The model under review builds one solid part; all positions refer to its coordinate system, in mm. A direction names the side the tool comes from. Coordinates: 2 decimals unless noted, no trailing zeros. Loops run counter-clockwise (first coordinate to the right, second up) from the corner with the lowest first, then second, coordinate; pieces in that order, holes last. Notation, with made-up numbers: M 52.25,28 L 86.25,28 A13 ccw 86.25,37 Z; hole C -7.75,57 d7. An arc over 180 degrees is marked long. Return JSON: item names as keys, results as strings.
```python
from build123d import *

# Parameters (mm, degrees)
SALIENTE_EXTRUIR1_DEPTH     = 46
CROQUIS3_W                  = 5
CROQUIS3_H                  = 17
CORTAR_EXTRUIR1_DEPTH       = 107
VACIADO1_T                  = -5
CORTAR_EXTRUIR3_DEPTH       = 5
CROQUIS7_W                  = 28.084979232
CROQUIS7_H                  = 13.64051807
CORTAR_EXTRUIR5_DEPTH       = 2
CROQUIS8_W                  = 84.286700134
CROQUIS8_H                  = 59.012293191
CORTAR_EXTRUIR6_DEPTH       = 50
CROQUIS9_W                  = 89.93795334
CROQUIS9_H                  = 8.49113686
CORTAR_EXTRUIR7_DEPTH       = 10
REDONDEO1_R                 = 2
REDONDEO2_R                 = 2
REDONDEO3_R                 = 2
CROQUIS10_W                 = 19.827227688
CROQUIS10_H                 = 42.140696998
CORTAR_EXTRUIR8_DEPTH       = 2
CROQUIS11_R                 = 2.017504942
CROQUIS11_R_2               = 1.891140859
CORTAR_EXTRUIR9_DEPTH       = 9
CROQUIS12_R                 = 2.25
CORTAR_EXTRUIR10_DEPTH      = 33
CORTAR_EXTRUIR11_START      = -3
CROQUIS13_R                 = 2.075
CORTAR_EXTRUIR11_DEPTH      = 7
CORTAR_EXTRUIR12_DEPTH      = 20
CORTAR_EXTRUIR12_DEPTH_BACK = 1
CORTAR_EXTRUIR12_START      = 10
CROQUIS14_R                 = 2.5
CROQUIS15_W                 = 7.96749323
CROQUIS15_H                 = 3.005999516
SALIENTE_EXTRUIR2_DEPTH     = 10
CROQUIS16_R                 = 1.5
CORTAR_EXTRUIR13_DEPTH      = 73
CROQUIS17_W                 = 124.159046256
CROQUIS17_H                 = 73.830112024
CORTAR_EXTRUIR14_DEPTH      = 2
CORTAR_EXTRUIR15_DEPTH      = 10
SALIENTE_EXTRUIR3_DEPTH     = 41
REDONDEO4_R                 = 10


with BuildPart() as part:
    # Croquis1 → Saliente-Extruir1 (new body)
    with BuildSketch(Plane.XY):
        Polygon((-50, -27.25), (-50, -29.825247619), (50, -29.825247619), (50, -27.25), (50, 27.25), (-50, 27.25), align=None)
    extrude(amount=SALIENTE_EXTRUIR1_DEPTH)

    # Croquis3 → Cortar-Extruir1 (cut)
    with BuildSketch(Plane.ZY.offset(50)):
        Polygon((46, 27.25), (5, 27.25), (11, 16.857695155), (46, 8.318575661), align=None)
        with Locations((2.5, 18.75)):
            Rectangle(CROQUIS3_W, CROQUIS3_H)
    extrude(amount=-CORTAR_EXTRUIR1_DEPTH, mode=Mode.SUBTRACT)

    # Vaciado1
    vaciado1_openings = [part.faces().sort_by_distance(p)[0] for p in [
        (0, -10.753335979, 46),
    ]]
    offset(amount=VACIADO1_T, openings=vaciado1_openings, kind=Kind.INTERSECTION)

    # Croquis5 → Cortar-Extruir3 (cut)
    with BuildSketch(Plane(origin=(0, 0, 0), x_dir=(-1, 0, 0), z_dir=(0, 0, -1))):
        Polygon((-44.96897667, -22.941518711), (-44.96897667, -34.965963837), (44.96897667, -34.965963837), (44.96897667, -22.941518711), (44.96897667, 22.941518711), (-44.96897667, 22.941518711), align=None)
    extrude(amount=-CORTAR_EXTRUIR3_DEPTH, mode=Mode.SUBTRACT)

    # Croquis7 → Cortar-Extruir5 (cut)
    with BuildSketch(Plane(origin=(0, 0, 0), x_dir=(-1, 0, 0), z_dir=(0, 0, -1))):
        Rectangle(CROQUIS7_W, CROQUIS7_H)
    extrude(amount=-CORTAR_EXTRUIR5_DEPTH, mode=Mode.SUBTRACT)

    # Croquis8 → Cortar-Extruir6 (cut)
    with BuildSketch(Plane(origin=(0, 0, 2), x_dir=(-1, 0, 0), z_dir=(0, 0, -1))):
        with Locations((0, -42.853406707)):
            Rectangle(CROQUIS8_W, CROQUIS8_H)
    extrude(amount=-CORTAR_EXTRUIR6_DEPTH, mode=Mode.SUBTRACT)

    # Croquis9 → Cortar-Extruir7 (cut)
    with BuildSketch(Plane(origin=(0, 0, 5), x_dir=(-1, 0, 0), z_dir=(0, 0, -1))):
        with Locations((0, 9.49556843)):
            Rectangle(CROQUIS9_W, CROQUIS9_H)
    extrude(amount=-CORTAR_EXTRUIR7_DEPTH, mode=Mode.SUBTRACT)

    # Redondeo1
    redondeo1_edges = [part.edges().sort_by_distance(p)[0] for p in [
        (-50, -29.825247619, 23),
        (42.143350067, -29.825247619, 25.5),
    ]]
    fillet(redondeo1_edges, radius=REDONDEO1_R)

    # Redondeo2
    redondeo2_edges = [part.edges().sort_by_distance(p)[0] for p in [
        (50, -29.825247619, 23),
    ]]
    fillet(redondeo2_edges, radius=REDONDEO2_R)

    # Redondeo3
    redondeo3_edges = [part.edges().sort_by_distance(p)[0] for p in [
        (-42.143350067, -29.825247619, 25.5),
    ]]
    fillet(redondeo3_edges, radius=REDONDEO3_R)

    # Croquis10 → Cortar-Extruir8 (cut)
    with BuildSketch(Plane(origin=(0, 13.586066701, 3.314658486), x_dir=(1, 0, 0), z_dir=(0, -0.9715041436001179, -0.237022570587279))):
        with Locations((13.913613844, 22.867026133)):
            Rectangle(CROQUIS10_W, CROQUIS10_H)
        with Locations((-13.913613844, 22.867026133)):
            Rectangle(CROQUIS10_W, CROQUIS10_H)
    extrude(amount=-CORTAR_EXTRUIR8_DEPTH, mode=Mode.SUBTRACT)

    # Croquis11 → Cortar-Extruir9 (cut)
    with BuildSketch(Plane(origin=(0, 0, 0), x_dir=(-1, 0, 0), z_dir=(0, 0, -1))):
        with Locations((-47, 14.614370501)):
            Circle(CROQUIS11_R)
        with Locations((47, 14.614370501)):
            Circle(CROQUIS11_R_2)
    extrude(amount=-CORTAR_EXTRUIR9_DEPTH, mode=Mode.SUBTRACT)

    # Croquis12 → Cortar-Extruir10 (cut)
    with BuildSketch(Plane(origin=(0, 0, 0), x_dir=(-1, 0, 0), z_dir=(0, 0, -1))):
        with Locations(Location((40, 20.614370501, 0), (0, 0, 90))):
            Circle(CROQUIS12_R)
        with Locations(Location((-40, 20.614370501, 0), (0, 0, 90))):
            Circle(CROQUIS12_R)
    extrude(amount=-CORTAR_EXTRUIR10_DEPTH, mode=Mode.SUBTRACT)

    # Croquis13 → Cortar-Extruir11 (cut)
    with BuildSketch(Plane(origin=(0, 0, 5), x_dir=(-1, 0, 0), z_dir=(0, 0, -1)).offset(CORTAR_EXTRUIR11_START)):
        with Locations(Location((47, 14.614370501, 0), (0, 0, 90))):
            Circle(CROQUIS13_R)
        with Locations(Location((-47, 14.614370501, 0), (0, 0, 37.647903634))):
            Circle(CROQUIS13_R)
    extrude(amount=-CORTAR_EXTRUIR11_DEPTH, mode=Mode.SUBTRACT)

    # Croquis14 → Cortar-Extruir12 (cut, two sides: drawn at the far end of the back side and taken through both)
    with BuildSketch(Plane(origin=(0, 0, 5), x_dir=(-1, 0, 0), z_dir=(0, 0, -1)).offset(CORTAR_EXTRUIR12_START - CORTAR_EXTRUIR12_DEPTH_BACK)):
        with Locations((-47, 14.614370501)):
            Circle(CROQUIS14_R)
        with Locations((47, 14.614370501)):
            Circle(CROQUIS14_R)
    extrude(amount=CORTAR_EXTRUIR12_DEPTH + CORTAR_EXTRUIR12_DEPTH_BACK, mode=Mode.SUBTRACT)

    # Croquis15 → Saliente-Extruir2 (add)
    with BuildSketch(Plane(origin=(0, 0, 15), x_dir=(-1, 0, 0), z_dir=(0, 0, -1))):
        with Locations((-40.985230055, 12.238137102)):
            Rectangle(CROQUIS15_W, CROQUIS15_H)
        with Locations((40.985230055, 12.238137102)):
            Rectangle(CROQUIS15_W, CROQUIS15_H)
    extrude(amount=SALIENTE_EXTRUIR2_DEPTH)

    # Croquis16 → Cortar-Extruir13 (cut)
    with BuildSketch(Plane(origin=(0, 0, 0), x_dir=(-1, 0, 0), z_dir=(0, 0, -1))):
        with Locations((-47.484488335, 5.25)):
            Circle(CROQUIS16_R)
        with Locations((-47.484488335, -20.75)):
            Circle(CROQUIS16_R)
        with Locations((-47.484488335, -7.75)):
            Circle(CROQUIS16_R)
        with Locations((47.484488335, -7.75)):
            Circle(CROQUIS16_R)
        with Locations((47.484488335, -20.75)):
            Circle(CROQUIS16_R)
        with Locations((47.484488335, 5.25)):
            Circle(CROQUIS16_R)
    extrude(amount=-CORTAR_EXTRUIR13_DEPTH, mode=Mode.SUBTRACT)

    # Croquis17 → Cortar-Extruir14 (cut)
    with BuildSketch(Plane(origin=(0, 0, 0), x_dir=(-1, 0, 0), z_dir=(0, 0, -1))):
        Rectangle(CROQUIS17_W, CROQUIS17_H)
    extrude(amount=-CORTAR_EXTRUIR14_DEPTH, mode=Mode.SUBTRACT)

    # Croquis19 → Cortar-Extruir15 (cut)
    with BuildSketch(Plane.XY.offset(8)):
        Polygon((47, 11.114370501), (50.031088913, 12.864370501), (50.031088913, 16.364370501), (47, 18.114370501), (43.968911087, 16.364370501), (43.968911087, 12.864370501), align=None)
        Polygon((-43.968911087, 12.864370501), (-47, 11.114370501), (-50.031088913, 12.864370501), (-50.031088913, 16.364370501), (-47, 18.114370501), (-43.968911087, 16.364370501), align=None)
    extrude(amount=CORTAR_EXTRUIR15_DEPTH, mode=Mode.SUBTRACT)

    # Croquis21 → Saliente-Extruir3 (add)
    with BuildSketch(Plane.XY.offset(46)):
        with BuildLine():
            Line((-22.763380433, 37.82435205), (-24.067061415, 32.609628124))
            Line((-24.067061415, 32.609628124), (-27.833250917, 28.463205933))
            Line((-27.833250917, 28.463205933), (-33.41481635, 8.318575661))
            Line((-33.41481635, 8.318575661), (-38.697259097, 8.318575661))
            add(Edge.make_bspline(
                [(-38.697259097, 8.318575661), (-39.050795871, 28.768789272), (-22.763380433, 37.82435205)],
                knots=[0, 0, 0, 1, 1, 1], degree=2))
        make_face()
        with BuildLine():
            Line((27.833250917, 28.463205933), (33.41481635, 8.318575661))
            Line((33.41481635, 8.318575661), (38.697259097, 8.318575661))
            add(Edge.make_bspline(
                [(38.697259097, 8.318575661), (39.050795871, 28.768789272), (22.763380433, 37.82435205)],
                knots=[0, 0, 0, 1, 1, 1], degree=2))
            Line((22.763380433, 37.82435205), (24.067061415, 32.609628124))
            Line((24.067061415, 32.609628124), (27.833250917, 28.463205933))
        make_face()
    extrude(amount=-SALIENTE_EXTRUIR3_DEPTH)

    # Redondeo4
    redondeo4_edges = [part.edges().sort_by_distance(p)[0] for p in [
        (-32.231829779, 12.588135408, 28.5),
        (32.231829779, 12.588135408, 28.5),
    ]]
    fillet(redondeo4_edges, radius=REDONDEO4_R)


solid = part.part
```
1. Add section C-C on z = 34. State how many separate pieces and enclosed holes the cut face has, plus the area to 3 significant figures.
Check values:
{"separate pieces": "1", "enclosed holes": "6", "area": "1,170 mm²"}
2. Insertion check: pin 1 Ø8 at (x, y) = (29.5, 30.5) entering from -Z; pin 2 Ø1.5 at (y, z) = (16, 33.5) entering from -X; pin 3 Ø1.4 at (x, z) = (-43.5, 21.5) entering from +Y; pin 4 Ø1.8 at (x, y) = (-47.48, -7.75) entering from +Z. Each pin has a flat end and moves straight along its axis. Give the tip position at first contact, or say it passes through.
Check values:
{"pin 1": "z = 5", "pin 2": "x = -38.29", "pin 3": "y = 14.47", "pin 4": "through"}
3. Machinability: for faces 1 (the face through (32.82, 10.47, 10.67)), 2 (the face through (42, 10.735, 10)), 3 (the face through (48.521, 17.236, 9.34)), 4 (the face through (-45.6, 13.1, 8)), which of the approach directions +Z, -Z, +X, -X, +Y, -Y give a long, thin tool a straight path to every point of the face, cutting with its end or side? Answer none if there is none.
Check values:
{"face 1": "-Z, -Y", "face 2": "-Z", "face 3": "+Z", "face 4": "none"}
4. Add section B-B on x = -40. Give the boundary of the cut face in (y, z).
Check values:
{"outline": "M 3.17,46 L 10.74,15 L 10.74,5 L 18.36,5 L 18.36,10.13 L 16.86,11 L 8.32,46 Z; M 22.86,5 L 27.25,5 L 22.86,7.53 Z"}
5. To check wall thickness, follow line 1 (X direction, y = -8, z = 11.5); line 2 (X direction, y = -19, z = 17); line 3 (Y direction, x = -47, z = 6.1). State the ranges of each line that lie inside material, in increasing order.
Check values:
{"line 1": "-50 to -48.96, -46.01 to -45, 45 to 46.01, 48.96 to 50", "line 2": "-50 to -45, 45 to 50", "line 3": "-29.83 to -22.17, -19.33 to -9.17, -6.33 to 3.83, 6.67 to 12.72, 16.51 to 25.34"}
6. The part is to be moulded in two halves that separate along Y. For faces 5 (the face through (-48.8, 15.2, 6.5)), 6 (the face through (36, 8.319, 15)), 7 (the face through (-50, -6, 24)), say which applies: released by +Y, released by -Y, zero draft, split by the parting line, or undercut.
Check values:
{"face 5": "undercut", "face 6": "released by -Y", "face 7": "zero draft"}
